Autodesk Inventor part; units mm, degrees
ref_plane "YZ Plane" through (0, 0, 0) normal (1, 0, 0) x (0, 1, 0)
ref_plane "XZ Plane" through (0, 0, 0) normal (0, 1, 0) x (-1, 0, 0)
ref_plane "XY Plane" through (0, 0, 0) normal (0, 0, 1) x (1, 0, 0)
sketch "Sketch1" plane through (0, 0, 0) normal (0, 0, 1) x (1, 0, 0)
  line L0 (0, 0) -> (92.58, 0)
  line L1 (92.58, 0) -> (92.58, 33.35)
  line L2 (92.58, 33.35) -> (-92.58, 33.35)
  line L3 (-92.58, 33.35) -> (-92.58, -33.35)
  line L4 (-92.58, -33.35) -> (92.58, -33.35)
  line L5 (92.58, -33.35) -> (92.58, 33.35)
  line L6 (-92.58, 33.35) -> (-89.58, 33.35)
  line L7 (-89.58, 33.35) -> (-89.58, 28.35)
  line L8 (92.58, -33.35) -> (89.58, -33.35)
  line L9 (89.58, -33.35) -> (89.58, -28.35)
  line L10 (-89.58, 28.35) -> (89.58, 28.35)
  line L11 (89.58, 28.35) -> (89.58, -28.35)
  line L12 (89.58, -28.35) -> (-89.58, -28.35)
  line L13 (-89.58, -28.35) -> (-89.58, 28.35)
  dimension "d0" = 92.58
  dimension "d1" = 33.35
  dimension "d2" = 185.16
  dimension "d3" = 66.7
  dimension "d4" = 3
  dimension "d5" = 5
  dimension "d6" = 3
  dimension "d7" = 5
extrude "Extrusion1" add sketch "Sketch1" along normal blind 2 contours L11 L10 L7 L2 L1 L0 | L0 L5 L4 L9 L11 | L9 L4 L3 L2 L7 L13 L12
sketch "Sketch2" plane through (-89.58, -28.35, 0) normal (0, 1, 0) x (1, 0, 0)
  line L0 (179.16, -2) -> (0, -2)
  line L1 (0, 0) -> (179.16, 0)
  line L2 (179.16, 0) -> (179.16, -2)
  line L3 (179.16, -2) -> (0, -2)
  line L4 (0, -2) -> (0, 0)
  point P0 (89.58, 0)
extrude "Extrusion2" cut sketch "Sketch2" against normal blind 1
sketch "Sketch3" plane through (0, 0, 2) normal (0, 0, 1) x (1, 0, 0)
  point P0 (0, 0)
sketch "Sketch4" plane through (0, 0, 2) normal (0, 0, 1) x (1, 0, 0)
  line L0 (92.58, -33.35) -> (92.58, 33.35)
  line L1 (92.58, 33.35) -> (99.58, 33.35)
  line L2 (99.58, 33.35) -> (99.58, -33.35)
  line L3 (99.58, -33.35) -> (92.58, -33.35)
  line L4 (89.58, 28.35) -> (89.58, -29.35)
  line L5 (89.58, -29.35) -> (96.58, -29.35)
  line L6 (96.58, -29.35) -> (96.58, 28.35)
  line L7 (96.58, 28.35) -> (89.58, 28.35)
  point P0 (0, 0)
  point P1 (92.58, 28.35)
  point P2 (92.58, -29.35)
  dimension "d12" = 7
  dimension "d13" = 90
  dimension "d14" = 7
  dimension "d15" = 90
extrude "Extrusion3" add sketch "Sketch4" against normal blind 2 contours L0 L5 L6 L7 L1 L2 L3
sketch "Sketch5" plane through (0, 0, 2) normal (0, 0, 1) x (1, 0, 0)
  line L0 (-89.58, 28.35) -> (89.58, 28.35)
  line L1 (96.58, -29.35) -> (92.58, -29.35)
  line L2 (89.58, 28.35) -> (92.58, 28.35)
  line L3 (92.58, 28.35) -> (92.58, -29.35)
  line L4 (92.58, -29.35) -> (89.58, -29.35)
  line L5 (89.58, -29.35) -> (89.58, 28.35)
  point P0 (0, 0)
extrude "Extrusion4" cut sketch "Sketch5" against normal blind 2
equation "\"d2\" = 2 * d0"
equation "\"d3\" = 2 * d1"
properties part number "Front cover"
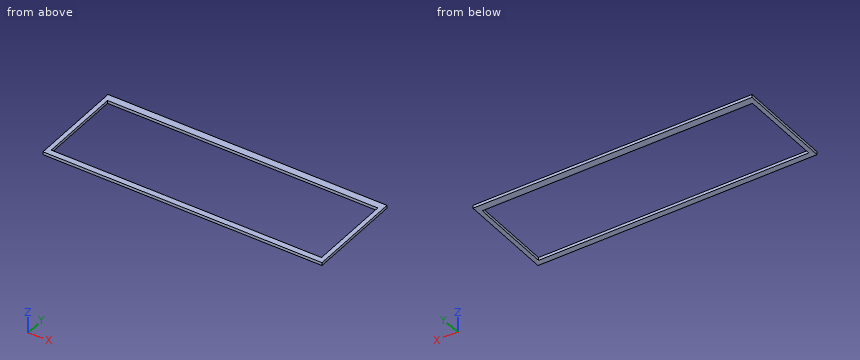
Here's how the part is built. I have some questions about the finished solid (model axes, mm). Coordinates: 2 decimals unless noted, no trailing zeros. Write each loop counter-clockwise with the first axis right and the second up, starting at its lowest first coordinate (ties: lowest second). Pieces come first, ordered by that corner, then holes.
1) If we section it at B-B (y = -18): List the corners of the cut face in (x, z) for me.
Filled in:
outline: (-92.58, 0) - (-89.58, 0) - (-89.58, 2) - (-92.58, 2) - close; (96.58, 0) - (99.58, 0) - (99.58, 2) - (96.58, 2) - close
2) If we section it at C-C (z = 1.2): List the corners of the cut face in (x, y) for me.
Filled in:
outline: (-92.58, -33.35) - (99.58, -33.35) - (99.58, 33.35) - (-92.58, 33.35) - close; hole (-89.58, -29.35) - (96.58, -29.35) - (96.58, 28.35) - (-89.58, 28.35) - close
3) If we section it at A-A (x = 28.5): List the corners of the cut face in (y, z) for me.
Filled in:
outline: (-33.35, 0) - (-29.35, 0) - (-29.35, 2) - (-33.35, 2) - close; (28.35, 0) - (33.35, 0) - (33.35, 2) - (28.35, 2) - close
4) If I drill on line 1 (X direction, y = 9.5, z = 0.9); line 2 (Y direction, x = -13, z = 1.35), over which ranges is the centre line in solid material (lowest first)?
Filled in:
line 1: x = -92.58 to -89.58, 96.58 to 99.58
line 2: y = -33.35 to -29.35, 28.35 to 33.35
